Verification items for the finished model (mm, model axes). Round coordinates to 2 decimals unless told otherwise and drop trailing zeros. Loops run counter-clockwise (first coordinate to the right, second up) from the corner with the lowest first, then second, coordinate; pieces in that order, holes last. Notation, with made-up numbers: M 79,64 L 137,64 A14 cw 137,90 Z; hole C 61.25,-33.75 d7. An arc over 180 degrees is marked long. Write item = value, one per line. Start each with the question number.
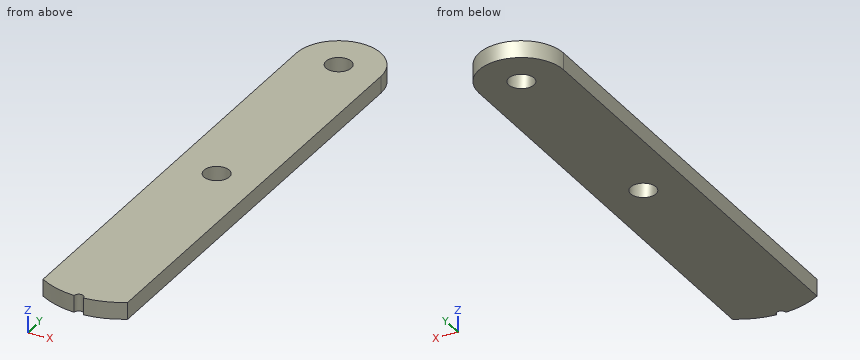
from build123d import *

# Parameters (mm, degrees)
SKETCH1_R           = 1.5
BOSS_EXTRUDE1_DEPTH = 2
SKETCH2_R           = 0.550401242
CUT_EXTRUDE1_DEPTH  = 10


with BuildPart() as part:
    # Sketch1 → Boss-Extrude1 (new body)
    with BuildSketch(Plane.XY):
        with BuildLine():
            Line((-5, 24.5), (-5, -29.5))
            ThreePointArc((-5, -29.5), (0, -30.913706536), (5, -29.5))
            Line((5, -29.5), (5, 24.5))
            ThreePointArc((5, 24.5), (0, 29.5), (-5, 24.5))
        make_face()
        with Locations((0, 24.5)):
            Circle(SKETCH1_R, mode=Mode.SUBTRACT)
        with Locations((0, -1.5)):
            Circle(SKETCH1_R, mode=Mode.SUBTRACT)
    extrude(amount=BOSS_EXTRUDE1_DEPTH)

    # Sketch2 → Cut-Extrude1 (cut)
    with BuildSketch(Plane.XY.offset(2)):
        with Locations((0, -30.913706536)):
            Circle(SKETCH2_R)
    extrude(amount=-CUT_EXTRUDE1_DEPTH, mode=Mode.SUBTRACT)


solid = part.part
1. Thickness scan on line 1 (Y direction, x = 0, z = 1); line 2 (Y direction, x = -1, z = 1.2); line 3 (Y direction, x = -4, z = 0.9). Record the ranges inside material, lowest first.
2. Gauge pin test, flat ends, axial feed: P1, Ø2.5, axis at x = 0, y = 24.5, coming from the +Z side; P2, Ø4, axis at x = -3, y = 17.5, coming from the -Z side. Record the tip position at first contact, or that the pin passes through.
3. Section check B-B, the plane y = -1.5. Enter the section's corners in (x, z), and give its area (3 significant figures).
4. Section check A-A, the plane x = 0. Enter the section's corners in (y, z).
5. Section check D-D, the plane x = 2.75. Enter the section's corners in (y, z), and give its area (3 significant figures).
6. Section check C-C, the plane z = 0.65. Enter the section's corners in (x, y).
Computed values:
q1.line_1 = -30.36 to -3, 0 to 23, 26 to 29.5
q1.line_2 = -30.86 to -2.62, -0.38 to 23.38, 25.62 to 29.4
q1.line_3 = -30.04 to 27.5
q2.P1 = through
q2.P2 = 0
q3.outline = M -5,0 L -1.5,0 L -1.5,2 L -5,2 Z; M 1.5,0 L 5,0 L 5,2 L 1.5,2 Z
q3.area = 14.0 mm2
q4.outline = M -30.36,0 L -3,0 L -3,2 L -30.36,2 Z; M 0,0 L 23,0 L 23,2 L 0,2 Z; M 26,0 L 29.5,0 L 29.5,2 L 26,2 Z
q5.outline = M -30.51,0 L 28.68,0 L 28.68,2 L -30.51,2 Z
q5.area = 118 mm2
q6.outline = M -5,-29.5 A9.55 ccw -0.55,-30.9 A0.55 cw 0.55,-30.9 A9.55 ccw 5,-29.5 L 5,24.5 A5 ccw -5,24.5 Z; hole C 0,-1.5 d3; hole C 0,24.5 d3
